from build123d import *

# Parameters (mm, degrees)
BOSS_EXTRUDE1_DEPTH = 40.1
SKETCH3_R           = 9
SKETCH2_R           = 11
CUT_EXTRUDE1_START  = -37.5
CUT_EXTRUDE1_DEPTH  = 37.5
SKETCH6_R           = 2.05
CUT_EXTRUDE2_DEPTH  = 2.6
SKETCH7_R           = 2.5
BOSS_EXTRUDE2_DEPTH = 14
WRAP4_START         = -32.470653403
WRAP4_DEPTH         = 8.340653403
CUT_EXTRUDE4_DEPTH  = 8.340653
CUT_EXTRUDE5_DEPTH  = 14


# Read off the part's stored shape, not the designer's step: Wrap4
with BuildPart() as part:
    # Sketch1 → Boss-Extrude1 (new body)
    with BuildSketch(Plane.XY):
        with BuildLine():
            Line((26.5, 5.25), (20.333162568, 5.25))
            ThreePointArc((20.333162568, 5.25), (0, 21), (-20.333162568, 5.25))
            Line((-20.333162568, 5.25), (-26.5, 5.25))
            ThreePointArc((-26.5, 5.25), (-31.75, 0), (-26.5, -5.25))
            Line((-26.5, -5.25), (-20.333162568, -5.25))
            ThreePointArc((-20.333162568, -5.25), (0, -21), (20.333162568, -5.25))
            Line((20.333162568, -5.25), (26.5, -5.25))
            ThreePointArc((26.5, -5.25), (31.75, 0), (26.5, 5.25))
        make_face()
    extrude(amount=-BOSS_EXTRUDE1_DEPTH)

    # Sketch3 → Loft1 section 0
    with BuildSketch(Plane.XY.offset(2)):
        Circle(SKETCH3_R)
    # Sketch2 → Loft1 section 1
    with BuildSketch(Plane.XY):
        Circle(SKETCH2_R)
    loft()

    # Sketch4 → Cut-Extrude1 (cut)
    with BuildSketch(Plane(origin=(0, 0, -40.1), x_dir=(-1, 0, 0), z_dir=(0, 0, -1)).offset(CUT_EXTRUDE1_START)):
        with BuildLine():
            Line((-26.5, 5.25), (-20.333162568, 5.25))
            ThreePointArc((-20.333162568, 5.25), (-21, 0), (-20.333162568, -5.25))
            Line((-20.333162568, -5.25), (-26.5, -5.25))
            ThreePointArc((-26.5, -5.25), (-31.75, 0), (-26.5, 5.25))
        make_face()
        with BuildLine():
            Line((26.5, -5.25), (20.333162568, -5.25))
            ThreePointArc((20.333162568, -5.25), (21, 0), (20.333162568, 5.25))
            Line((20.333162568, 5.25), (26.5, 5.25))
            ThreePointArc((26.5, 5.25), (31.75, 0), (26.5, -5.25))
        make_face()
    extrude(amount=CUT_EXTRUDE1_DEPTH, mode=Mode.SUBTRACT)

    # Sketch6 → Cut-Extrude2 (cut)
    with BuildSketch(Plane.XY):
        with Locations((-26.5, 0)):
            Circle(SKETCH6_R)
        with Locations(Location((26.5, 0, 0), (0, 0, 180))):
            Circle(SKETCH6_R)
    extrude(amount=-CUT_EXTRUDE2_DEPTH, mode=Mode.SUBTRACT)

    # Sketch7 → Boss-Extrude2 (add)
    with BuildSketch(Plane.XY.offset(2)):
        Circle(SKETCH7_R)
    extrude(amount=BOSS_EXTRUDE2_DEPTH)

    # Wrap4 outline → Wrap4 (add)
    with BuildSketch(Plane.XY.offset(WRAP4_START)):
        with BuildLine():
            ThreePointArc((-20.9308697, -1.702555024), (-18.186533479, 10.5), (-8.990978947, 18.977942396))
            Line((-8.990978947, 18.977942396), (-16.269390476, 34.341038621))
            ThreePointArc((-16.269390476, 34.341038621), (-32.908965344, 19), (-37.874907076, -3.080813854))
            Line((-37.874907076, -3.080813854), (-20.9308697, -1.702555024))
        make_face()
    extrude(amount=WRAP4_DEPTH)

    # Sketch19 → Cut-Extrude4 (cut)
    with BuildSketch(Plane(origin=(0, 0, -32.470653403), x_dir=(-1, 0, 0), z_dir=(0, 0, -1))):
        with BuildLine():
            Line((16.269390476, 34.341038621), (37.874907076, -3.080813854))
            ThreePointArc((37.874907076, -3.080813854), (32.908965344, 19), (16.269390476, 34.341038621))
        make_face()
    extrude(amount=-CUT_EXTRUDE4_DEPTH, mode=Mode.SUBTRACT)

    # Sketch20 → Cut-Extrude5 (cut)
    with BuildSketch(Plane(origin=(0, 0, -32.470653403), x_dir=(-1, 0, 0), z_dir=(0, 0, -1))):
        Polygon((16.269390476, 34.341038621), (8.990978947, 18.977942396), (21.1022034, 25.970361093), align=None)
        Polygon((37.874907076, -3.080813854), (20.9308697, -1.702555024), (33.042094152, 5.289863673), align=None)
    extrude(amount=-CUT_EXTRUDE5_DEPTH, mode=Mode.SUBTRACT)


solid = part.part
Verification items for the finished model (mm, model axes). A direction names the side the tool comes from. Give positions to 0.01 mm unless a question says otherwise; leave off trailing zeros. Order: outer loops, then holes, each group sorted by start corner. A loop starts at its lowest first (then second) coordinate and runs counter-clockwise, first axis right, second up. Notation, with made-up numbers: (31, 47) -> (73, 47) arc R15 cw to (73, 56) -> close; hole circle Ø6 at (-26, 75). An arc over 180 degrees is marked (long way). Answer as CSV lines item,"result".
Q1. Scan lines: probe 1 along Z at (x, y) = (21, -4.5); probe 2 along Z at (x, y) = (-14.5, 21); probe 3 along Y at (x, z) = (26.5, -0.7). Record each from-to range of solid material in increasing order.
Solutions:
probe 1,"z = -2.6 to 0"
probe 2,"z = -32.47 to -24.13"
probe 3,"y = -5.25 to -2.05, 2.05 to 5.25"
Q2. Sectioned sample at B-B on z = -26. Record the cut outline in (x, y).
Solutions:
outline,"(-33.04, 5.29) -> (-20.93, -1.7) arc R21 ccw (long way) to (-8.99, 18.98) -> (-21.1, 25.97) -> close"
Q3. Access from +Z, -Z, +X, -X, +Y, -Y to the whole of each face (thin tool, end or side, straight path). Record for faces 1 (the cylindrical face through (-31.75, 0.12, -1.28)), 2 (the flat face through (-23, -5.25, -1)), 3 (the flat face through (2, -2, 2)), 4 (the flat face through (-21, 12, -32.471)).
Solutions:
face 1,"+Z, -X"
face 2,"+Z, -Z, -X, -Y"
face 3,"+Z"
face 4,"-Z, -X, +Y"
Q4. Sectioned sample at C-C on y = 0. Count the separate pieces of the cut face and the enclosed holes in it, plus the area to 3 significant figures.
Solutions:
separate pieces,"3"
enclosed holes,"0"
area,"1,850 mm²"
Q5. Sectioned sample at A-A on x = 0. Record the cut outline in (y, z), plus the area to 3 significant figures.
Solutions:
outline,"(-21, -40.1) -> (21, -40.1) -> (21, 0) -> (11, 0) -> (9, 2) -> (2.5, 2) -> (2.5, 16) -> (-2.5, 16) -> (-2.5, 2) -> (-9, 2) -> (-11, 0) -> (-21, 0) -> close"
area,"1,790 mm²"
Q6. Release check for a two-part mould opening along Y. For faces 5 (the cylindrical face through (-28.55, 0.09, -1.28)), 6 (the flat face through (-8, -9, 0)), 7 (the cylindrical face through (-0.54, -2.44, 8.9)) record: +Y half, -Y half, draft (parallel to the pull), parting line (faces both ways), or undercut.
Solutions:
face 5,"undercut"
face 6,"draft"
face 7,"parting line"
Q7. Depth check by flat-ended pin: pin 1 (1.5 mm diameter, centred on x = 2.5, y = 5.5, fed in from +Z); pin 2 (3.5 mm diameter, centred on x = -26.5, y = 0, fed in from -Z); pin 3 (1.3 mm diameter, centred on x = 25, z = -2, fed in from +Y). Enter the tip coordinate at first touch or a pass-through.
Solutions:
pin 1,"stops at z = 2"
pin 2,"stops at z = -32.47"
pin 3,"stops at y = 5.25"
Q8. Sectioned sample at D-D on z = 5. Record the cut outline in (x, y), plus the area to 3 significant figures.
Solutions:
outline,"circle Ø5 at (0, 0)"
area,"19.6 mm²"
